Work out the finished part from the listing and answer in its coordinate system (mm). A direction names the side the tool comes from. Coordinates: 2 decimals unless noted, no trailing zeros. Write each loop counter-clockwise with the first axis right and the second up, starting at its lowest first coordinate (ties: lowest second). Pieces come first, ordered by that corner, then holes. Notation, with made-up numbers: (34.5, 20) - (80.5, 20) arc R25 cw to (80.5, 46) - close; hole circle Ø3 at (56, 34). An arc over 180 degrees is marked (long way). One line per item, written item: value.
Autodesk Fusion 360 part; units mm, degrees
sketch "Sketch1" plane through (0, 0, 0) normal (0, 1, 0) x (1, 0, 0)
  line L0 (45, 22.5) -> (-45, 22.5)
  line L1 (-45, 22.5) -> (-45, -22.5)
  line L2 (-45, -22.5) -> (45, -22.5)
  line L3 (45, -22.5) -> (45, 22.5)
  line L4 (45, 22.5) -> (-45, -22.5) construction
  line L5 (-45, 22.5) -> (45, -22.5) construction
  dimension "d1" = 45
  dimension "d2" = 90
extrude "Extrude1" add sketch "Sketch1" along normal blind 4
sketch "Sketch2" plane through (0, 0, -22.5) normal (0, 0, -1) x (-1, 0, 0)
  line L0 (45, 0) -> (-45, 0)
  line L1 (-45, 0) -> (-45, 45)
  line L2 (-45, 45) -> (45, 45)
  line L3 (45, 45) -> (45, 0)
  point P0 (-45, 0)
  point P1 (45, 0)
  dimension "d12" = 45
extrude "Extrude4" add sketch "Sketch2" against normal blind 4
sketch "Sketch3" plane through (-45, 0, 0) normal (-1, 0, 0) x (0, 0, 1)
  line L0 (-22.5, 0) -> (22.5, 0)
  line L1 (22.5, 0) -> (22.5, 4)
  line L2 (22.5, 4) -> (-18.5, 4)
  line L3 (-22.5, 45) -> (-22.5, 0)
  line L4 (-18.5, 45) -> (-18.5, 4)
  line L5 (22.5, 4) -> (-18.5, 45)
  line L6 (-18.5, 4) -> (-18.5, 45)
  line L7 (-18.5, 45) -> (-22.5, 45)
extrude "Extrude3" add sketch "Sketch3" against normal blind 4 contours L2 L4 L5 L6
mirror "Mirror1" about plane through (0, 0, 0) normal (1, 0, 0) of "Extrude3"
sketch "Sketch4" plane through (0, 0, -18.5) normal (0, 0, 1) x (1, 0, 0)
  line L0 (41, 4) -> (41, 45)
  line L1 (41, 45) -> (-41, 45)
  line L2 (-41, 45) -> (-41, 4)
  line L3 (-41, 4) -> (41, 4)
  circle A0 centre (-22.5, 22.5) radius 3.25
  line L4 (-22.5, 22.5) -> (-16, 22.5) construction
  line L5 (45, 45) -> (-45, 45)
  line L6 (-45, 0) -> (45, 0)
  line L7 (0, 0) -> (0, 21) construction
  circle A1 centre (22.5, 22.5) radius 3.25
  dimension "d15" = 6.5
  dimension "d16" = 45
extrude "Extrude5" cut sketch "Sketch4" against normal through all contours A0 | A1
sketch "Sketch5" plane through (0, 0, 0) normal (0, -1, 0) x (1, 0, 0)
  line L0 (45, -22.5) -> (45, 22.5)
  line L1 (45, 22.5) -> (-45, 22.5)
  line L2 (-45, 22.5) -> (-45, -22.5)
  line L3 (-45, -22.5) -> (45, -22.5)
  circle A0 centre (-25, 2.5) radius 6.25
  line L4 (18.25, 12.25) -> (31.75, 12.25)
  line L5 (31.75, 12.25) -> (31.75, -7.25)
  line L6 (31.75, -7.25) -> (18.25, -7.25)
  line L7 (18.25, -7.25) -> (18.25, 12.25)
  line L8 (-25, 2.5) -> (31.5002, 2.5) construction
  line L9 (-45, -22.5) -> (45, -22.5)
  line L10 (25, -13) -> (25, 19) construction
  line L11 (-25, 2.5) -> (-25, -11) construction
  line L12 (0, 0) -> (0, -11) construction
  circle A1 centre (-6, 2.5) radius 2.5
  circle A2 centre (6, 2.5) radius 2.5
  dimension "d18" = 12.5
  dimension "d19" = 19.5
  dimension "d20" = 13.5
  dimension "d21" = 25
  dimension "d22" = 50
  dimension "d26" = 5
  dimension "d27" = 12
extrude "Extrude6" cut sketch "Sketch5" against normal blind 4 contours A0 | L4 L5 L6 L7 | A1 | A2
chamfer "Chamfer1" distance 2 angle 45 2 edges at (25, 4, -7.25) (25, 4, 12.25)
Item 1: Which of the six approach directions +Z, -Z, +X, -X, +Y, -Y give full straight-line access (tool end or side, diameter ignored) to faces 1 (the face through (25, 1, -7.25)), 2 (the face through (25.09, 2.99, -8.24)), 3 (the face through (41, 16, -7))?
Evaluation:
face 1: +Y, -Y
face 2: +Y
face 3: +Z, +Y
Item 2: Section B-B, the plane y = 22.5 is taken. Determine the outline of the cut face in (x, z).
Evaluation:
outline: (-45, -22.5) - (-25.75, -22.5) - (-25.75, -18.5) - (-41, -18.5) - (-41, 4) - (-45, 4) - close; (-19.25, -22.5) - (19.25, -22.5) - (19.25, -18.5) - (-19.25, -18.5) - close; (25.75, -22.5) - (45, -22.5) - (45, 4) - (41, 4) - (41, -18.5) - (25.75, -18.5) - close
Item 3: Section D-D, the plane z = 16 is taken. Determine the outline of the cut face in (x, y), then the cut area to 3 significant figures.
Evaluation:
outline: (-45, 0) - (45, 0) - (45, 10.5) - (41, 10.5) - (41, 4) - (-41, 4) - (-41, 10.5) - (-45, 10.5) - close
area: 412 mm2
Item 4: Section A-A, the plane x = 22.5 is taken. Determine the outline of the cut face in (y, z).
Evaluation:
outline: (0, -22.5) - (19.25, -22.5) - (19.25, -18.5) - (4, -18.5) - (4, -9.25) - (2, -7.25) - (0, -7.25) - close; (0, 12.25) - (2, 12.25) - (4, 14.25) - (4, 22.5) - (0, 22.5) - close; (25.75, -22.5) - (45, -22.5) - (45, -18.5) - (25.75, -18.5) - close
Item 5: Given pin 1 (12.5 mm diameter, centred on x = -17.5, z = 6, fed in from +Y); pin 2 (20.5 mm diameter, centred on x = -11, y = 14.5, fed in from +Z), each flat-ended and moving along its own axis, determine where each tip first touches the part or whether it passes through.
Evaluation:
pin 1: stops at y = 4
pin 2: stops at z = -18.5
Item 6: Consider probe 1 along X at (y, z) = (5.5, 14.5); probe 2 along Z at (x, y) = (-6, 0.95); probe 3 along X at (y, z) = (22, -20). Determine where each line is inside the solid, lowest interval first.
Evaluation:
probe 1: x = -45 to -41, 41 to 45
probe 2: z = -22.5 to 0, 5 to 22.5
probe 3: x = -45 to -25.71, -19.29 to 19.29, 25.71 to 45
Item 7: Section C-C, the plane x = 6 is taken. Determine the outline of the cut face in (y, z).
Evaluation:
outline: (0, -22.5) - (45, -22.5) - (45, -18.5) - (4, -18.5) - (4, 0) - (0, 0) - close; (0, 5) - (4, 5) - (4, 22.5) - (0, 22.5) - close
Item 8: Determine the mould class of faces 4 (the face through (-43, 24.2, 2.3)), 5 (the face through (25, 1, 12.25)), 6 (the face through (45, 18, -5)) for opening direction X: +X half, -X half, draft (parallel to the pull), parting line (faces both ways), or undercut.
Evaluation:
face 4: draft
face 5: undercut
face 6: +X half
